from build123d import *

# Parameters (mm, degrees)
SKETCH2_W          = 81.219896545
SKETCH2_H          = 40.203731022
CUT_EXTRUDE1_DEPTH = 35
CUT_EXTRUDE2_DEPTH = 35
SKETCH4_R          = 9.5
CUT_EXTRUDE3_DEPTH = 569.968860373


with BuildPart() as part:
    # Sketch1 → Revolve1 (revolve)
    with BuildSketch(Plane.XY, mode=Mode.PRIVATE) as revolve1_sk:
        Polygon((0, 0), (575, 0), (575, 30), (200, 22), (0, 22), align=None)
    revolve1 = revolve(revolve1_sk.sketch.rotate(Axis((0, 0, 0), (1, 0, 0)), 90), axis=Axis((0, 0, 0), (1, 0, 0)))

    # Sketch2 → Cut-Extrude1 (cut, symmetric)
    with BuildSketch(Plane.XY):
        with Locations((555.609948272, 30.101865511)):
            Rectangle(SKETCH2_W, SKETCH2_H)
        with Locations((555.609948272, -30.101865511)):
            Rectangle(SKETCH2_W, SKETCH2_H)
    cut_extrude1 = extrude(amount=CUT_EXTRUDE1_DEPTH, both=True, mode=Mode.SUBTRACT)

    # Sketch3 → Cut-Extrude2 (cut, symmetric)
    with BuildSketch(Plane(origin=(0, 10, 0), x_dir=(1, 0, 0), z_dir=(0, 1, 0))):
        with BuildLine():
            Line((515, 26.922823032), (540, 26.922823032))
            ThreePointArc((540, 26.922823032), (566.922823032, 0), (540, -26.922823032))
            Line((540, -26.922823032), (515, -26.922823032))
            Line((515, -26.922823032), (515, -33.426109463))
            Line((515, -33.426109463), (579.528771991, -33.426109463))
            Line((579.528771991, -33.426109463), (579.528771991, 35.099670457))
            Line((579.528771991, 35.099670457), (515, 35.099670457))
            Line((515, 35.099670457), (515, 26.922823032))
        make_face()
    cut_extrude2 = extrude(amount=CUT_EXTRUDE2_DEPTH, both=True, mode=Mode.SUBTRACT)

    # Sketch4 → Cut-Extrude3 (cut, through all)
    with BuildSketch(Plane(origin=(0, 10, 0), x_dir=(1, 0, 0), z_dir=(0, 1, 0))):
        with Locations(Location((540, 0, 0), (0, 0, 180))):
            Circle(SKETCH4_R)
    cut_extrude3 = extrude(amount=-CUT_EXTRUDE3_DEPTH, mode=Mode.SUBTRACT)

    # Mirror1: Revolve1, Cut-Extrude1, Cut-Extrude2, Cut-Extrude3 across plane
    add(revolve1.mirror(Plane(origin=(0, 0, 0), x_dir=(0, 0, 1), z_dir=(1, 0, 0))))
    add(cut_extrude1.mirror(Plane(origin=(0, 0, 0), x_dir=(0, 0, 1), z_dir=(1, 0, 0))), mode=Mode.SUBTRACT)
    add(cut_extrude2.mirror(Plane(origin=(0, 0, 0), x_dir=(0, 0, 1), z_dir=(1, 0, 0))), mode=Mode.SUBTRACT)
    add(cut_extrude3.mirror(Plane(origin=(0, 0, 0), x_dir=(0, 0, 1), z_dir=(1, 0, 0))), mode=Mode.SUBTRACT)


solid = part.part
Read the model definition and answer for the solid it produces. Units are mm, in the model's axes. A direction names the side the tool comes from. Coordinates: 2 decimals unless noted, no trailing zeros. Write each loop counter-clockwise with the first axis right and the second up, starting at its lowest first coordinate (ties: lowest second). Pieces come first, ordered by that corner, then holes. Notation, with made-up numbers: (64.5, 11.5) -> (89.5, 11.5) arc R16 cw to (89.5, 26.5) -> close; hole circle Ø5 at (12.25, -15.75). An arc over 180 degrees is marked (long way). Return JSON: item names as keys, results as strings.
(1) The part is cut by section A-A on z = 0. Give the vertices of the cut face in (x, y).
Answers below:
{"outline": "(-566.92, -10) -> (-549.5, -10) -> (-549.5, 10) -> (-566.92, 10) -> close; (-530.5, -10) -> (-515, -10) -> (-515, -28.72) -> (-200, -22) -> (200, -22) -> (515, -28.72) -> (515, -10) -> (530.5, -10) -> (530.5, 10) -> (515, 10) -> (515, 28.72) -> (200, 22) -> (-200, 22) -> (-515, 28.72) -> (-515, 10) -> (-530.5, 10) -> close; (549.5, -10) -> (566.92, -10) -> (566.92, 10) -> (549.5, 10) -> close"}
(2) Each of these flat-tipped pins is pushed along its axis until it touches: P1, Ø15.5, axis at x = 541, z = -12, coming from the -Y side; P2, Ø6, axis at y = 13.5, z = 3.5, coming from the +X side; P3, Ø5, axis at y = -4, z = 10.5, coming from the +X side. Where does it stop, or does it pass through?
Answers below:
{"P1": "y = -10", "P2": "x = 515", "P3": "x = 565.71"}
(3) The part is cut by section D-D on x = 404.5. Give the vertices of the cut face in (y, z).
Answers below:
{"outline": "circle Ø52.73 at (0, 0)"}
(4) Which of the six approach directions +Z, -Z, +X, -X, +Y, -Y give full straight-line access (tool end or side, diameter ignored) to faces 1 (the flat face through (-528, 0, 26.923)), 2 (the flat face through (-529, 10, 0)), 3 (the flat face through (-529, -10, 0)), 4 (the conical face through (355.29, 15.4, -20.09))?
Answers below:
{"face 1": "+Z, -X, +Y, -Y", "face 2": "+Z, -Z, -X, +Y", "face 3": "+Z, -Z, -X, -Y", "face 4": "none"}
(5) The part is cut by section C-C on x = 13. Give the vertices of the cut face in (y, z), then the cut area to 3 significant figures.
Answers below:
{"outline": "circle Ø44 at (0, 0)", "area": "1,520 mm^2"}
(6) For a pull along Z with two mould halves and no side action, classify faces 5 (the flat face through (527, 0, -26.923)), 6 (the cylindrical face through (-530.939, 0.14, 2.854)), 7 (the flat face through (528, 0, 26.923)) as pulls with the +Z half, pulls with the -Z half, needs draft (parallel to the pull), parting line crosses it, or undercut.
Answers below:
{"face 5": "pulls with the -Z half", "face 6": "undercut", "face 7": "pulls with the +Z half"}
(7) The part is cut by section B-B on y = 0. Give the vertices of the cut face in (x, z).
Answers below:
{"outline": "(-540, -26.92) -> (-515, -26.92) -> (-515, -28.72) -> (-200, -22) -> (200, -22) -> (515, -28.72) -> (515, -26.92) -> (540, -26.92) arc R26.92 ccw to (540, 26.92) -> (515, 26.92) -> (515, 28.72) -> (200, 22) -> (-200, 22) -> (-515, 28.72) -> (-515, 26.92) -> (-540, 26.92) arc R26.92 ccw to start; hole circle Ø19 at (-540, 0); hole circle Ø19 at (540, 0)"}
(8) Consider line 1 along Z through (x, y) = (540, 4); line 2 along X through (y, z) = (3, -2); line 3 along X through (y, z) = (-5.5, 6.5). Determine where each line is inside the solid, lowest interval first. Write a range as from..to.
Answers below:
{"line 1": "-26.92..-9.5, 9.5..26.92", "line 2": "-566.85..-549.29, -530.71..530.71, 549.29..566.85", "line 3": "-566.13..-546.93, -533.07..533.07, 546.93..566.13"}
